Build history of the part. All positions in model axes, mm. A direction names the side the tool comes from. Give positions to 0.01 mm unless a question says otherwise; leave off trailing zeros. Order: outer loops, then holes, each group sorted by start corner. A loop starts at its lowest first (then second) coordinate and runs counter-clockwise, first axis right, second up. Notation, with made-up numbers: M -31,-3.5 L -5,-3.5 A13 ccw -5,5.5 Z; hole C -36,32.25 d2. An arc over 180 degrees is marked long. Use CSV: the item, a comma, the result in double quotes. Start each with the question number.
Item 1: Which spindle directions (+Z, -Z, +X, -X, +Y, -Y) get a long thin tool onto all of the face, cutting with end or side? Do faces 1 (the flat face through (34, -29, 3)), 2 (the flat face through (6.595, -2.465, -37.402)), 3 (the flat face through (6.6, -2.46, 37.44)), 4 (the cylindrical face through (36.493, -2.465, 0.713)). Say none if no direction does.
Item 2: Band-saw the part on A-A on x = 12. Write the cut outline in (y, z), plus the area to 3 significant figures.
Item 3: Pin check, flat tips, straight feed: P1, Ø4, axis at y = -22.5, z = -8, coming from the +X side; P2, Ø2, axis at y = -30.5, z = 22.5, coming from the +X side; P3, Ø4, axis at y = -20, z = -0.5, coming from the -X side. Stop position of each tip, or through.
Item 4: Two-plate mould, pull along Z, no slides. Class faces 5 (the flat face through (0, -27, 37)), 6 (the flat face through (6.595, -52.535, 37.402)), 7 (the cylindrical face through (34.49, -39.65, -0.76)): pulls with the +Z half, pulls with the -Z half, needs draft (parallel to the pull), parting line crosses it, or undercut.
Item 5: Band-saw the part on C-C on y = -36.5. Write the cut outline in (x, z), plus the area to 3 significant figures.
Item 6: Band-saw the part on D-D on x = 28. Write the cut outline in (y, z), plus the area to 3 significant figures.
Item 7: Band-saw the part on B-B on z = 0. Write the cut outline in (x, y), plus the area to 3 significant figures.
Item 8: Wall check: line 1 along Z through (x, y) = (28.5, -23); line 2 along Z through (x, y) = (12, -45.5); line 3 along Y through (x, z) = (30, -19.5). Give the ranges that are in metal, low to high.
from build123d import *

# Parameters (mm, degrees)
F1_DEPTH = 55
F3_DEPTH = 5
F5_DEPTH = 5
F6_R     = 34.5
F6_R_2   = 33.5
F7_DEPTH = 26


with BuildPart() as f1:
    # F0 (on Front) → F1 (new body)
    with BuildSketch(Plane.XZ):
        with BuildLine():
            Line((0, -33.5), (0, -39.5))
            ThreePointArc((0, -39.5), (39.5, 0), (0, 39.5))
            Line((0, 39.5), (0, 33.5))
            ThreePointArc((0, 33.5), (33.5, 0), (0, -33.5))
        make_face()
    extrude(amount=F1_DEPTH)

    # F2 (on face) → F3 (cut)
    with BuildSketch(Plane.XZ.offset(55)):
        with BuildLine():
            Line((6.859103, -38.899906), (6.338158, -35.945483))
            ThreePointArc((6.338158, -35.945483), (36.5, 0), (6.338158, 35.945483))
            Line((6.338158, 35.945483), (6.859103, 38.899906))
            ThreePointArc((6.859103, 38.899906), (3.442652, 39.349691), (0, 39.5))
            Line((0, 39.5), (0, 33.5))
            ThreePointArc((0, 33.5), (33.5, 0), (0, -33.5))
            Line((0, -33.5), (0, -39.5))
            ThreePointArc((0, -39.5), (3.442652, -39.349691), (6.859103, -38.899906))
        make_face()
    extrude(amount=-F3_DEPTH, mode=Mode.SUBTRACT)

    # F4 (on face) → F5 (cut)
    with BuildSketch(Plane(origin=(0, 0, 0), x_dir=(-1, 0, 0), z_dir=(0, 1, 0))):
        with BuildLine():
            Line((-6.859103, 38.899906), (-6.338158, 35.945483))
            ThreePointArc((-6.338158, 35.945483), (-36.5, 0), (-6.338158, -35.945483))
            Line((-6.338158, -35.945483), (-6.859103, -38.899906))
            ThreePointArc((-6.859103, -38.899906), (-3.442652, -39.349691), (0, -39.5))
            Line((0, -39.5), (0, -33.5))
            ThreePointArc((0, -33.5), (-33.5, 0), (0, 33.5))
            Line((0, 33.5), (0, 39.5))
            ThreePointArc((0, 39.5), (-3.442652, 39.349691), (-6.859103, 38.899906))
        make_face()
    extrude(amount=-F5_DEPTH, mode=Mode.SUBTRACT)

    # F6 (on face) → F7 (cut)
    with BuildSketch(Plane.XZ.offset(55)):
        Circle(F6_R)
        Circle(F6_R_2, mode=Mode.SUBTRACT)
    extrude(amount=-F7_DEPTH, mode=Mode.SUBTRACT)


solid = f1.part
Model answer:
1,face 1,"-X, -Y"
1,face 2,"-Z, -X, +Y"
1,face 3,"+Z, -X, +Y"
1,face 4,"-X, +Y"
2,outline,"M -55,-37.63 L 0,-37.63 L 0,-34.47 L -5,-34.47 L -5,-31.28 L -29,-31.28 L -29,-32.35 L -50,-32.35 L -50,-34.47 L -55,-34.47 Z; M -55,34.47 L -50,34.47 L -50,32.35 L -29,32.35 L -29,31.28 L -5,31.28 L -5,34.47 L 0,34.47 L 0,37.63 L -55,37.63 Z"
2,area,"590 mm^2"
3,P1,"stops at x = 39.04"
3,P2,"stops at x = 33.14"
3,P3,"stops at x = 33.41"
4,face 5,"needs draft"
4,face 6,"pulls with the +Z half"
4,face 7,"undercut"
5,outline,"M 0,-39.5 A39.5 ccw 0,39.5 L 0,34.5 A34.5 cw 0,-34.5 Z"
5,area,"581 mm^2"
6,outline,"M -55,-27.86 L 0,-27.86 L 0,-23.41 L -5,-23.41 L -5,-18.39 L -29,-18.39 L -29,-20.16 L -50,-20.16 L -50,-23.41 L -55,-23.41 Z; M -55,23.41 L -50,23.41 L -50,20.16 L -29,20.16 L -29,18.39 L -5,18.39 L -5,23.41 L 0,23.41 L 0,27.86 L -55,27.86 Z"
6,area,"867 mm^2"
7,outline,"M 33.5,-29 L 34.5,-29 L 34.5,-50 L 36.5,-50 L 36.5,-55 L 39.5,-55 L 39.5,0 L 36.5,0 L 36.5,-5 L 33.5,-5 Z"
7,area,"279 mm^2"
8,line 1,"z = -27.35 to -17.61, 17.61 to 27.35"
8,line 2,"z = -37.63 to -32.35, 32.35 to 37.63"
8,line 3,"y = -50 to -5"
